Here's how the part is built. I have some questions about the finished solid (model axes, mm). Round coordinates to 2 decimals unless told otherwise and drop trailing zeros. Order: outer loops, then holes, each group sorted by start corner. A loop starts at its lowest first (then second) coordinate and runs counter-clockwise, first axis right, second up. Notation, with made-up numbers: M 56,-19 L 83,-19 A20 cw 83,0 Z; hole C -16,24.25 d7. An arc over 180 degrees is marked long. Use one line per item in the form item = value. Start each with the question number.
```python
from build123d import *

# Parameters (mm, degrees)
SKETCH2_W           = 65
SKETCH2_H           = 35
BOSS_EXTRUDE1_DEPTH = 0.3
SKETCH3_R           = 1.75
CUT_EXTRUDE1_DEPTH  = 1.6
SKETCH4_R           = 3.25
SKETCH4_R_2         = 1.75
BOSS_EXTRUDE2_DEPTH = 1.5
CUT_EXTRUDE2_DEPTH  = 10


with BuildPart() as part:
    # Sketch2 → Boss-Extrude1 (new body)
    with BuildSketch(Plane.XY):
        Rectangle(SKETCH2_W, SKETCH2_H)
    extrude(amount=BOSS_EXTRUDE1_DEPTH)

    # Sketch3 → Cut-Extrude1 (cut)
    with BuildSketch(Plane.XY.offset(0.3)):
        with Locations((-28.5, 13.5)):
            Circle(SKETCH3_R)
        with Locations((-28.5, -13.5)):
            Circle(SKETCH3_R)
        with Locations((22.5, 13.5)):
            Circle(SKETCH3_R)
        with Locations((22.5, -13.5)):
            Circle(SKETCH3_R)
    extrude(amount=-CUT_EXTRUDE1_DEPTH, mode=Mode.SUBTRACT)

    # Sketch4 → Boss-Extrude2 (add)
    with BuildSketch(Plane.XY.offset(0.3)):
        with Locations((-28.5, 13.5)):
            Circle(SKETCH4_R)
        with Locations((-28.5, 13.5)):
            Circle(SKETCH4_R_2, mode=Mode.SUBTRACT)
        with Locations((-28.5, -13.5)):
            Circle(SKETCH4_R)
        with Locations((-28.5, -13.5)):
            Circle(SKETCH4_R_2, mode=Mode.SUBTRACT)
        with Locations((22.5, -13.5)):
            Circle(SKETCH4_R)
        with Locations((22.5, -13.5)):
            Circle(SKETCH4_R_2, mode=Mode.SUBTRACT)
        with Locations((22.5, 13.5)):
            Circle(SKETCH4_R)
        with Locations((22.5, 13.5)):
            Circle(SKETCH4_R_2, mode=Mode.SUBTRACT)
    extrude(amount=BOSS_EXTRUDE2_DEPTH)

    # Sketch5 → Cut-Extrude2 (cut)
    with BuildSketch(Plane.XY.offset(0.3)):
        with BuildLine():
            Line((-32.5, 6.75), (-26.5, 6.75))
            ThreePointArc((-26.5, 6.75), (-18.75, -1), (-26.5, -8.75))
            Line((-26.5, -8.75), (-32.5, -8.75))
            ThreePointArc((-32.5, -8.75), (-40.25, -1), (-32.5, 6.75))
        make_face()
    extrude(amount=-CUT_EXTRUDE2_DEPTH, mode=Mode.SUBTRACT)


solid = part.part
```
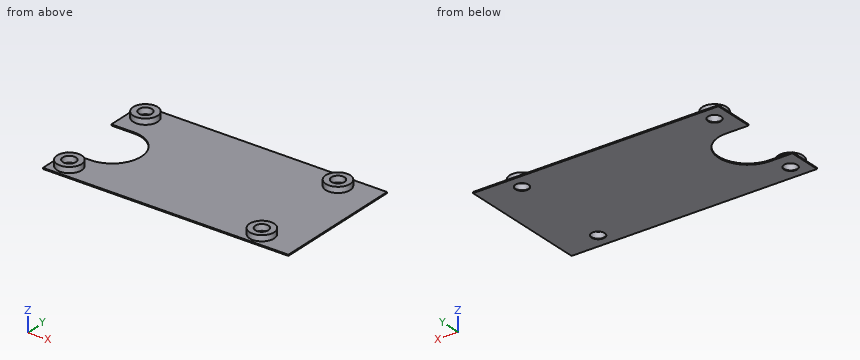
1) If we section it at B-B on x = 22.5: Write out the boundary of the cut face in (y, z), then the cut area to 3 significant figures.
2) Will these pins go through, and if not, where does the flat tip stop? pin 1 Ø3 at (x, y) = (22.5, 13.5) entering from -Z; pin 2 Ø10.5 at (x, y) = (4.5, 4.5) entering from +Z.
3) If I drill on line 1 (Y direction, x = -28.5, z = 0.95); line 2 (Y direction, x = 22.5, z = 0.2); line 3 (Y direction, x = -28.5, z = 0.1), over which ranges is the centre line in solid material (lowest first)?
4) If we section it at D-D on x = -23.5: Write out the boundary of the cut face in (y, z), then the cut area to 3 significant figures.
5) If we section it at C-C on y = 13.5: Write out the boundary of the cut face in (x, z), then the cut area to 3 significant figures.
6) If we section it at A-A on z = 1.15: Write out the boundary of the cut face in (x, y), then the cut area to 3 significant figures.
Completed:
q1.outline = M -17.5,0 L -15.25,0 L -15.25,1.8 L -16.75,1.8 L -16.75,0.3 L -17.5,0.3 Z; M -11.75,0 L 11.75,0 L 11.75,1.8 L 10.25,1.8 L 10.25,0.3 L -10.25,0.3 L -10.25,1.8 L -11.75,1.8 Z; M 15.25,0 L 17.5,0 L 17.5,0.3 L 16.75,0.3 L 16.75,1.8 L 15.25,1.8 Z
q1.area = 17.4 mm²
q2.pin_1 = through
q2.pin_2 = 0.3
q3.line_1 = -16.75 to -15.25, -11.75 to -10.25, 10.25 to 11.75, 15.25 to 16.75
q3.line_2 = -17.5 to -15.25, -11.75 to 11.75, 15.25 to 17.5
q3.line_3 = -17.5 to -15.25, -11.75 to -8.75, 6.75 to 11.75, 15.25 to 17.5
q4.outline = M -17.5,0 L -8.15,0 L -8.15,0.3 L -17.5,0.3 Z; M 6.15,0 L 17.5,0 L 17.5,0.3 L 6.15,0.3 Z
q4.area = 6.21 mm²
q5.outline = M -32.5,0 L -30.25,0 L -30.25,1.8 L -31.75,1.8 L -31.75,0.3 L -32.5,0.3 Z; M -26.75,0 L 20.75,0 L 20.75,1.8 L 19.25,1.8 L 19.25,0.3 L -25.25,0.3 L -25.25,1.8 L -26.75,1.8 Z; M 24.25,0 L 32.5,0 L 32.5,0.3 L 25.75,0.3 L 25.75,1.8 L 24.25,1.8 Z
q5.area = 26.4 mm²
q6.outline = C -28.5,-13.5 d6.5; C -28.5,13.5 d6.5; C 22.5,-13.5 d6.5; C 22.5,13.5 d6.5; hole C -28.5,-13.5 d3.5; hole C -28.5,13.5 d3.5; hole C 22.5,-13.5 d3.5; hole C 22.5,13.5 d3.5
q6.area = 94.2 mm²
